The listing builds one solid part. Answer for the finished solid, in the listing's coordinates (mm). A direction names the side the tool comes from. Round coordinates to 2 decimals unless told otherwise and drop trailing zeros. Write each loop counter-clockwise with the first axis right and the second up, starting at its lowest first coordinate (ties: lowest second). Pieces come first, ordered by that corner, then holes. Notation, with made-up numbers: (7.25, 73) - (15.25, 73) arc R22 ccw to (15.25, 97) - close; hole circle Ø11 at (72.5, 49). An arc over 180 degrees is marked (long way). Return JSON: item names as keys, results as strings. Group by question number.
from build123d import *

# Parameters (mm, degrees)
F1_DEPTH = 12.7
F2_R     = 0.8957594025
F3_DEPTH = 2.54
F4_R     = 0.9017
F5_DEPTH = 25.4
F5_TAPER = -0.5
F7_DEPTH = 1.27


with BuildPart() as f1:
    # F0 (on Front) → F1 (new body)
    with BuildSketch(Plane.XZ):
        Polygon((-45.7861032019, -14.4099961261), (-45.5484393347, -18.2125762878), (-17.9987344891, -18.2125762878), (-17.9987344891, -14.4099961261), align=None)
        with BuildLine():
            ThreePointArc((-45.5484393347, -31.0462834481), (-50.3102929013, -24.629429868), (-45.5484393347, -18.2125762878))
            Line((-45.5484393347, -18.2125762878), (-45.7861032019, -14.4099961261))
            ThreePointArc((-45.7861032019, -14.4099961261), (-54.0189585577, -24.6331397871), (-45.7861032019, -34.8562834481))
            Line((-45.7861032019, -34.8562834481), (-45.5484393347, -31.0462834481))
        make_face()
        Polygon((-14.3427420408, -31.0462834481), (-45.5484393347, -31.0462834481), (-45.7861032019, -34.8562834481), (-14.3427420408, -34.8562834481), align=None)
    extrude(amount=F1_DEPTH)

    # F2 (on face) → F3 (join)
    with BuildSketch(Plane.YZ.offset(-17.9987344891)):
        with Locations((-6.3440594025, -16.3135261769)):
            Circle(F2_R)
    extrude(amount=F3_DEPTH)

    # F4 (on Right) → F5 (cut)
    with BuildSketch(Plane.YZ):
        with Locations((-6.35, -32.9512834481)):
            Circle(F4_R)
    extrude(amount=-F5_DEPTH, taper=F5_TAPER, mode=Mode.SUBTRACT)

    # F6 (on face) → F7 (join)
    with BuildSketch(Plane.XY.offset(-14.4099961261)):
        Polygon((-42.1013459563, -3.627152415), (-43.6947904527, -3.4279720858), (-39.6447889507, -10.731250979), (-37.7193801105, -10.731250979), (-34.6652828157, -6.2828902155), (-32.0759378374, -6.2828902155), (-29.3538048863, -10.731250979), (-26.6980677843, -10.731250979), (-23.2456084341, -3.627152415), (-25.1710172743, -3.627152415), (-27.6113765675, -8.6486606188), (-29.0882308036, -8.6486606188), (-31.3543434693, -4.9455032606), (-35.9267555177, -4.9455032606), (-37.7264208984, -8.6486606188), (-39.9767570198, -8.6486606188), align=None)
    extrude(amount=F7_DEPTH)


solid = f1.part
(1) Flat-ended cylindrical pins translate along their axes: pin 1 (0.6 mm diameter, centred on x = -24, z = -14, fed in from +Y); pin 2 (0.9 mm diameter, centred on y = -6.5, z = -16.5, fed in from +X); pin 3 (0.6 mm diameter, centred on x = -39.5, z = -14, fed in from +Y). Find the tip coordinate at first contact, or state that the pin passes through.
(2) Find section A-A (x = -28.5). Write down the section's boundary in (y, z), plus the area to 3 significant figures.
(3) For faces 1 (the flat face through (-34, -4.946, -14)), 2 (the flat face through (-30, -6, -31.046)), 3 (the flat face through (-24, -3.627, -14)), 4 (the flat face through (-28, -10.731, -14)), determine the directions among +Z, -Z, +X, -X, +Y, -Y from which every point of the face is accessible in a straight line to the end or side of a thin tool.
(4) Determine the mould class of faces 5 (the flat face through (-34.5, -12.7, -31.3)), 6 (the cylindrical face through (-50.31, -6.26, -24.75)), 7 (the flat face through (-30.73, -8.48, -13.78)) for opening direction X: +X half, -X half, draft (parallel to the pull), parting line (faces both ways), or undercut.
(5) Consider line 1 (Z direction, x = -43.5, y = -10.25); line 2 (Z direction, x = -31, y = -6.5); line 3 (Z direction, x = -23, y = -7). Determine where each line is inside the solid, lowest interval first.
(6) Find section C-C (z = -28.5). Write down the section's boundary in (x, y), plus the area to 3 significant figures.
(7) Find section D-D (y = -10.25). Write down the section's boundary in (x, z), plus the area to 3 significant figures.
(8) Find section B-B (y = -2.5). Write down the section's boundary in (x, z).
Check sheet entries:
{
 "1": {"pin 1": "stops at y = -3.63", "pin 2": "stops at x = -15.46", "pin 3": "stops at y = -8.65"},
 "2": {"outline": "(-12.7, -34.86) - (0, -34.86) - (0, -31.05) - (-12.7, -31.05) - close; (-12.7, -18.21) - (0, -18.21) - (0, -14.41) - (-8.65, -14.41) - (-8.65, -13.14) - (-10.73, -13.14) - (-10.73, -14.41) - (-12.7, -14.41) - close", "area": "99.3 mm^2"},
 "3": {"face 1": "+Z, +Y", "face 2": "+X, +Y, -Y", "face 3": "+Z, +X, +Y", "face 4": "+Z, +X, -X, -Y"},
 "4": {"face 5": "draft", "face 6": "+X half", "face 7": "undercut"},
 "5": {"line 1": "z = -34.86 to -31.05, -18.21 to -14.41", "line 2": "z = -34.86 to -31.05, -18.21 to -13.14", "line 3": "z = -34.86 to -33.84, -32.06 to -31.05, -18.21 to -14.41"},
 "6": {"outline": "(-53.28, -12.7) - (-49.08, -12.7) - (-49.08, 0) - (-53.28, 0) - close", "area": "53.3 mm^2"},
 "7": {"outline": "(-45.79, -34.86) - (-14.34, -34.86) - (-14.34, -31.05) - (-45.55, -31.05) arc R6.7 cw to (-45.55, -18.21) - (-18, -18.21) - (-18, -14.41) - (-26.46, -14.41) - (-26.46, -13.14) - (-29.65, -13.14) - (-29.65, -14.41) - (-37.39, -14.41) - (-37.39, -13.14) - (-39.91, -13.14) - (-39.91, -14.41) - (-45.79, -14.41) arc R10.46 ccw to start", "area": "316 mm^2"},
 "8": {"outline": "(-45.79, -34.86) - (-14.34, -34.86) - (-14.34, -31.05) - (-45.55, -31.05) arc R6.7 cw to (-45.55, -18.21) - (-18, -18.21) - (-18, -14.41) - (-45.79, -14.41) arc R10.46 ccw to start"}
}
